The drawing under review shows one solid part. Ordinate dimensions are in mm from its lowest x, y, z. Give positions to 0.01 mm unless a question says otherwise; leave off trailing zeros. Order: outer loops, then holes, each group sorted by start corner. A loop starts at its lowest first (then second) coordinate and runs counter-clockwise, first axis right, second up. Notation, with made-up numbers: (57, 13) -> (62, 13) arc R7 ccw to (62, 21) -> close; hole circle Ø1 at (6.5, 33.5). An arc over 180 degrees is marked (long way). One line per item, written item: value. Start each with the question number.
1) Consider section A-A (x = 58). State the section outline as (y, z) points, plus the area to 3 significant figures.
2) Consider section C-C (z = 4). State the section outline as (x, y) points.
3) For pin 1 (4 mm diameter, centred on x = 52, y = 5.5, fed in from -Z); pin 2 (3.5 mm diameter, centred on x = 65.5, z = 81, fed in from -Y); pin 3 (12 mm diameter, centred on x = 51.5, z = 70, fed in from -Y); pin 4 (2.5 mm diameter, centred on x = 58, z = 4, fed in from -Y), all flat-tipped, find the tip position at first contact; note any pin that passes through.
4) Consider section D-D (x = 18.5). State the section outline as (y, z) points.
5) Wall thickness on line 1 along X through (y, z) = (6.45, 81); line 2 along X through (y, z) = (3, 23.5); line 3 along Y through (x, z) = (39, 70): over which ranges is each line inside the solid? List them lowest first. Write a range as from..to.
6) The part is to be moulded in two halves that separate along Z. For the marked faces 1 and 2, say which applies: released by +Z, released by -Z, zero draft, split by the parting line, or undercut.
7) Consider section B-B (z = 64). State the section outline as (x, y) points, plus the area to 3 significant figures.
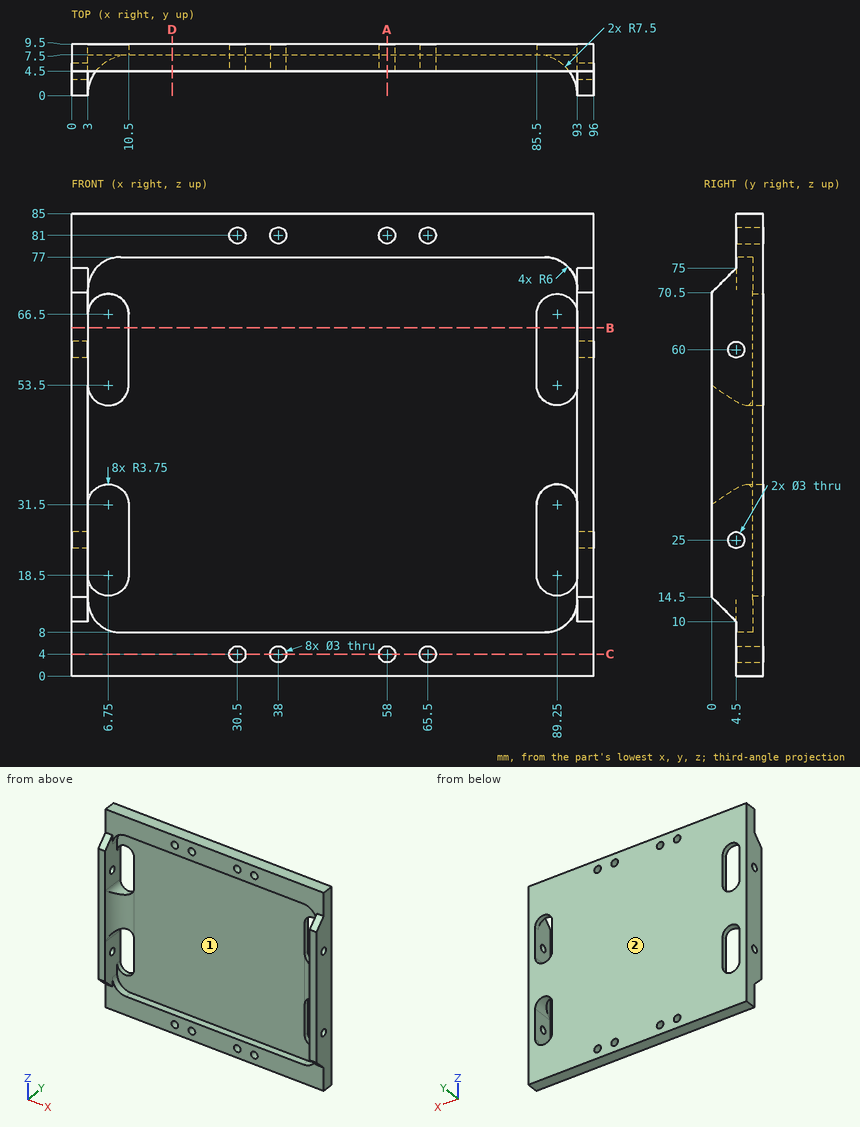
Checked values:
1. outline: (4.5, 0) -> (9.5, 0) -> (9.5, 2.5) -> (4.5, 2.5) -> close; (4.5, 5.5) -> (9.5, 5.5) -> (9.5, 79.5) -> (4.5, 79.5) -> (4.5, 77) -> (7.5, 77) -> (7.5, 8) -> (4.5, 8) -> close; (4.5, 82.5) -> (9.5, 82.5) -> (9.5, 85) -> (4.5, 85) -> close
1. area: 188 mm^2
2. outline: (0, 4.5) -> (29, 4.5) -> (29, 9.5) -> (0, 9.5) -> close; (32, 4.5) -> (36.5, 4.5) -> (36.5, 9.5) -> (32, 9.5) -> close; (39.5, 4.5) -> (56.5, 4.5) -> (56.5, 9.5) -> (39.5, 9.5) -> close; (59.5, 4.5) -> (64, 4.5) -> (64, 9.5) -> (59.5, 9.5) -> close; (67, 4.5) -> (96, 4.5) -> (96, 9.5) -> (67, 9.5) -> close
3. pin 1: stops at z = 0
3. pin 2: stops at y = 4.5
3. pin 3: stops at y = 7.5
3. pin 4: passes through
4. outline: (4.5, 0) -> (9.5, 0) -> (9.5, 85) -> (4.5, 85) -> (4.5, 77) -> (7.5, 77) -> (7.5, 8) -> (4.5, 8) -> close
5. line 1: x = 0..29, 32..36.5, 39.5..56.5, 59.5..64, 67..96
5. line 2: x = 0..3, 93..96
5. line 3: y = 7.5..9.5
6. face 1: undercut
6. face 2: zero draft
7. outline: (0, 0) -> (3, 0) -> (3, 9.5) -> (0, 9.5) -> close; (10.5, 7.5) -> (85.5, 7.5) -> (85.5, 9.5) -> (10.5, 9.5) -> close; (93, 0) -> (96, 0) -> (96, 9.5) -> (93, 9.5) -> close
7. area: 207 mm^2
